Verification items for the finished model (mm, model axes). A direction names the side the tool comes from. Give positions to 0.01 mm unless a question says otherwise; leave off trailing zeros. Loops run counter-clockwise (first coordinate to the right, second up) from the corner with the lowest first, then second, coordinate; pieces in that order, holes last. Notation, with made-up numbers: M 54.5,48 L 67.5,48 A20 ccw 67.5,54 Z; hole C 0.25,63.5 d4. An arc over 180 degrees is marked long. Answer in a Markdown table with one row per item.
```python
from build123d import *

# Parameters (mm, degrees)
SKETCH1_R           = 4.25
BOSS_EXTRUDE1_DEPTH = 6
SKETCH3_R           = 1.5
CUT_EXTRUDE1_DEPTH  = 7


with BuildPart() as part:
    # Sketch1 → Boss-Extrude1 (new body)
    with BuildSketch(Plane.XY):
        with BuildLine():
            Line((711, 350.5), (711, 385))
            ThreePointArc((711, 385), (708.071067812, 392.071067812), (701, 395))
            Line((701, 395), (681, 395))
            ThreePointArc((681, 395), (673.928932188, 392.071067812), (671, 385))
            Line((671, 385), (671, 310))
            ThreePointArc((671, 310), (673.928932188, 302.928932188), (681, 300))
            Line((681, 300), (701, 300))
            ThreePointArc((701, 300), (708.071067812, 302.928932188), (711, 310))
            Line((711, 310), (711, 344.5))
            Line((711, 344.5), (691, 344.5))
            Line((691, 344.5), (691, 350.5))
            Line((691, 350.5), (711, 350.5))
        make_face()
        with Locations((691, 310)):
            Circle(SKETCH1_R, mode=Mode.SUBTRACT)
        with Locations((691, 385)):
            Circle(SKETCH1_R, mode=Mode.SUBTRACT)
    extrude(amount=BOSS_EXTRUDE1_DEPTH)

    # Sketch3 → Cut-Extrude1 (cut, through all)
    with BuildSketch(Plane.XY.offset(6)):
        with Locations((691, 350.5)):
            Circle(SKETCH3_R)
        with Locations((691, 344.5)):
            Circle(SKETCH3_R)
    extrude(amount=-CUT_EXTRUDE1_DEPTH, mode=Mode.SUBTRACT)


solid = part.part
```
Item 1: Sectioned sample at C-C (x = 688). Record the cut outline in (y, z), and give its area (3 significant figures).
Reported:
| item | result |
|---|---|
| outline | M 300,0 L 306.99,0 L 306.99,6 L 300,6 Z; M 313.01,0 L 381.99,0 L 381.99,6 L 313.01,6 Z; M 388.01,0 L 395,0 L 395,6 L 388.01,6 Z |
| area | 498 mm^2 |
Item 2: Sectioned sample at D-D (x = 675). Record the cut outline in (y, z), and give its area (3 significant figures).
Reported:
| item | result |
|---|---|
| outline | M 302,0 L 393,0 L 393,6 L 302,6 Z |
| area | 546 mm^2 |
Item 3: Go/stop test with flat-tipped pins: pin 1 (1.8 mm diameter, centred on x = 704.5, z = 2, fed in from -Y); pin 2 (2.5 mm diameter, centred on y = 347.5, z = 2, fed in from +X); pin 3 (2 mm diameter, centred on x = 706, z = 5.5, fed in from +Y). Record where each tip stops, or that it passes through.
Reported:
| item | result |
|---|---|
| pin 1 | stops at y = 300.34 |
| pin 2 | stops at x = 691 |
| pin 3 | stops at y = 394.17 |
Item 4: Tool access check on faces 4 (the cylindrical face through (708.15, 391.99, 2.96)), 5 (the flat face through (702, 344.5, 3)). Record the directions out of +Z, -Z, +X, -X, +Y, -Y that give a thin tool (end or side, any length) a straight path to the whole face; none if there is none.
Reported:
| item | result |
|---|---|
| face 4 | +Z, -Z, +X, +Y |
| face 5 | +Z, -Z, +X |
Item 5: Sectioned sample at B-B (x = 704). Record the cut outline in (y, z).
Reported:
| item | result |
|---|---|
| outline | M 300.46,0 L 344.5,0 L 344.5,6 L 300.46,6 Z; M 350.5,0 L 394.54,0 L 394.54,6 L 350.5,6 Z |
Item 6: Sectioned sample at A-A (z = 3.8). Record the cut outline in (x, y).
Reported:
| item | result |
|---|---|
| outline | M 671,310 A10 ccw 681,300 L 701,300 A10 ccw 711,310 L 711,344.5 L 692.5,344.5 A1.5 cw long 691,346 L 691,349 A1.5 cw long 692.5,350.5 L 711,350.5 L 711,385 A10 ccw 701,395 L 681,395 A10 ccw 671,385 Z; hole C 691,310 d8.5; hole C 691,385 d8.5 |
Item 7: Scan lines: L1, parallel to Y at x = 690.5, z = 3.95; L2, parallel to Y at x = 699, z = 4.9; L3, parallel to X at y = 385, z = 3.3. Record each from-to range of solid material in increasing order. Write a range as [from, to].
Reported:
| item | result |
|---|---|
| L1 | y = [300, 305.78], [314.22, 343.09], [345.91, 349.09], [351.91, 380.78], [389.22, 395] |
| L2 | y = [300, 344.5], [350.5, 395] |
| L3 | x = [671, 686.75], [695.25, 711] |
Item 8: Release check for a two-part mould opening along X. For faces 1 (the cylindrical face through (673.85, 303.01, 2.96)), 2 (the flat face through (702, 350.5, 3)), 3 (the cylindrical face through (689.905, 343.475, 3.042)) record: released by +X, released by -X, zero draft, split by the parting line, or undercut.
Reported:
| item | result |
|---|---|
| face 1 | released by -X |
| face 2 | zero draft |
| face 3 | undercut |
